from build123d import *

# Parameters (mm, degrees)
F0_W     = 38.1
F0_H     = 6.35
F1_DEPTH = 6.35


with BuildPart() as f1:
    # F0 (on Right) → F1 (new body)
    with BuildSketch(Plane.YZ):
        Polygon((101.6, 38.1), (-101.6, 38.1), (-101.6, 12.7), (-107.95, 12.7), (-107.95, -19.05), (-101.6, -19.05), (-101.6, -38.1), (101.6, -38.1), (101.6, -19.05), (107.95, -19.05), (107.95, 12.7), (101.6, 12.7), align=None)
        with Locations((-50.8, -28.575)):
            Rectangle(F0_W, F0_H, mode=Mode.SUBTRACT)
        with Locations((50.8, -28.575)):
            Rectangle(F0_W, F0_H, mode=Mode.SUBTRACT)
    extrude(amount=F1_DEPTH)


solid = f1.part
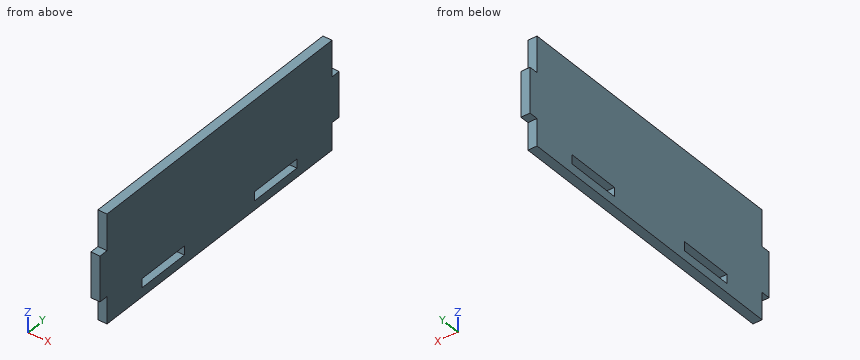
Verification items for the finished model (mm, model axes). Round coordinates to 2 decimals unless told otherwise and drop trailing zeros. Order: outer loops, then holes, each group sorted by start corner. A loop starts at its lowest first (then second) coordinate and runs counter-clockwise, first axis right, second up.
1. Section check C-C on z = -21. Record the cut outline in (x, y), then the cut area to 3 significant figures.
Final values:
outline: (0, -101.6) - (6.35, -101.6) - (6.35, 101.6) - (0, 101.6) - close
area: 1,290 mm2
2. Section check A-A on y = 54.5. Record the cut outline in (x, z).
Final values:
outline: (0, -38.1) - (6.35, -38.1) - (6.35, -31.75) - (0, -31.75) - close; (0, -25.4) - (6.35, -25.4) - (6.35, 38.1) - (0, 38.1) - close
3. Thickness scan on L1, parallel to Y at x = 5.25, z = -25.5; L2, parallel to Z at x = 2.5, y = -59.5; L3, parallel to Y at x = 1.25, z = -34. Record the ranges inside material, lowest first.
Final values:
L1: y = -101.6 to -69.85, -31.75 to 31.75, 69.85 to 101.6
L2: z = -38.1 to -31.75, -25.4 to 38.1
L3: y = -101.6 to 101.6
4. Go/stop test with flat-tipped pins: P1, Ø3, axis at x = 4.5, z = -27.5, coming from the -Y side; P2, Ø1.9, axis at x = 4, z = -27.5, coming from the +Y side; P3, Ø3, axis at x = 2, y = -103.5, coming from the +Z side. Record where each tip stops, or that it passes through.
Final values:
P1: stops at y = -101.6
P2: stops at y = 101.6
P3: stops at z = 12.7
5. Section check B-B on x = 2.5. Record the cut outline in (y, z), then the cut area to 3 significant figures.
Final values:
outline: (-107.95, -19.05) - (-101.6, -19.05) - (-101.6, -38.1) - (101.6, -38.1) - (101.6, -19.05) - (107.95, -19.05) - (107.95, 12.7) - (101.6, 12.7) - (101.6, 38.1) - (-101.6, 38.1) - (-101.6, 12.7) - (-107.95, 12.7) - close; hole (-69.85, -31.75) - (-31.75, -31.75) - (-31.75, -25.4) - (-69.85, -25.4) - close; hole (31.75, -31.75) - (69.85, -31.75) - (69.85, -25.4) - (31.75, -25.4) - close
area: 15,400 mm2
